Work out the finished part from the listing and answer in its coordinate system (mm). Round coordinates to 2 decimals unless told otherwise and drop trailing zeros. Order: outer loops, then holes, each group sorted by start corner. A loop starts at its lowest first (then second) coordinate and runs counter-clockwise, first axis right, second up. Notation, with made-up numbers: (-30, 55) -> (14, 55) arc R17 cw to (14, 70) -> close; hole circle Ø9 at (-39, 7.5). An arc over 180 degrees is marked (long way). Use one line per item in the form item = value.
```python
from build123d import *

# Parameters (mm, degrees)
SKETCH1_R           = 2.2225
BOSS_EXTRUDE1_DEPTH = 6.35


with BuildPart() as part:
    # Sketch1 → Boss-Extrude1 (new body)
    with BuildSketch(Plane(origin=(0, 0, 0), x_dir=(1, 0, 0), z_dir=(0, 1, 0))):
        with BuildLine():
            Line((-0.046089406, 3.174665457), (25.307821187, 3.542750442))
            ThreePointArc((25.307821187, 3.542750442), (38.709203085, 7.5965874), (47.926567326, 18.135601931))
            ThreePointArc((47.926567326, 18.135601931), (52.150559021, 19.658475583), (53.673432674, 15.434483888))
            ThreePointArc((53.673432674, 15.434483888), (42.151727371, 2.260715725), (25.4, -2.806580473))
            Line((25.4, -2.806580473), (0.046089406, -3.174665457))
            ThreePointArc((0.046089406, -3.174665457), (-3.174665457, -0.046089406), (-0.046089406, 3.174665457))
        make_face()
        with Locations(Location((0, 0, 0), (0, 0, 270))):
            Circle(SKETCH1_R, mode=Mode.SUBTRACT)
    extrude(amount=BOSS_EXTRUDE1_DEPTH)


solid = part.part
```
Item 1: Flat-ended cylindrical pins translate along their axes: P1, Ø2, axis at y = 4.5, z = -10, coming from the -X side; P2, Ø2, axis at x = 24.5, y = 4.5, coming from the -Z side; P3, Ø3, axis at x = 30.5, y = 2.5, coming from the -Z side. Find the tip coordinate at first contact, or state that the pin passes through.
Findings:
P1 = 40.67
P2 = -3.55
P3 = -4.54
Item 2: The part is cut by section D-D, the plane z = -13.5. Give the vertices of the cut face in (x, y), and give its area (3 significant figures).
Findings:
outline = (45.11, 0) -> (52.68, 0) -> (52.68, 6.35) -> (45.11, 6.35) -> close
area = 48.1 mm^2
Item 3: The part is cut by section C-C, the plane x = 20. Give the vertices of the cut face in (y, z), and give its area (3 significant figures).
Findings:
outline = (0, -3.47) -> (6.35, -3.47) -> (6.35, 2.88) -> (0, 2.88) -> close
area = 40.3 mm^2
Item 4: Determine the mould class of faces 1 (the flat face through (28, 0, -3)), 2 (the cylindrical face through (-2.17, 3.13, -0.48)), 3 (the cylindrical face through (38.54, 3.13, -7.49)), 4 (the cylindrical face through (42.36, 3.131, -2.396)) for opening direction Z: released by +Z, released by -Z, zero draft, split by the parting line, or undercut.
Findings:
face_1 = zero draft
face_2 = undercut
face_3 = released by -Z
face_4 = released by +Z
Item 5: Consider line 1 along X through (y, z) = (2.75, 0) (1 decimal); line 2 along X through (y, z) = (3.5, -0.25); line 3 along Z through (x, y) = (44, 3.75). Determine where each line is inside the solid, lowest interval first.
Findings:
line_1 = -3.2 to -2.2, 2.2 to 38
line_2 = -3.17 to -2.21, 2.21 to 38.54
line_3 = -12.15 to -3.55
